Could you check a few things on this model? Use its own coordinates, in mm. Round coordinates to 2 decimals unless told otherwise and drop trailing zeros. Loops run counter-clockwise (first coordinate to the right, second up) from the corner with the lowest first, then second, coordinate; pieces in that order, holes last. Notation, with made-up numbers: M -28,28 L -12,28 A16 ccw -12,48 Z; hole C 41,-32 d4. An arc over 180 degrees is marked long. Answer in a Markdown table with one row per item.
```python
from build123d import *

# Parameters (mm, degrees)
BOSS_EXTRUDE1_DEPTH         = 2.54
F_1_4_CLEARANCE_HOLE2_D     = 6.7564
F_1_4_CLEARANCE_HOLE2_DEPTH = 8.382
F_1_4_CLEARANCE_HOLE2_TIP   = 2.029827343


with BuildPart() as part:
    # Sketch1 → Boss-Extrude1 (new body)
    with BuildSketch(Plane(origin=(0, 0, 0), x_dir=(0, 0, -1), z_dir=(1, 0, 0))):
        with BuildLine():
            Line((6.35, -2.630256121), (6.35, -152.4))
            ThreePointArc((6.35, -152.4), (0, -158.75), (-6.35, -152.4))
            Line((-6.35, -152.4), (-6.35, 0))
            ThreePointArc((-6.35, 0), (-5.866635031, 2.430039796), (-4.490128061, 4.490128061))
            Line((-4.490128061, 4.490128061), (13.470384182, 22.450640303))
            ThreePointArc((13.470384182, 22.450640303), (22.450640303, 22.450640303), (22.450640303, 13.470384182))
            Line((22.450640303, 13.470384182), (6.35, -2.630256121))
        make_face()
    extrude(amount=BOSS_EXTRUDE1_DEPTH)

    # 1/4 Clearance Hole2
    with Locations(Plane(origin=(2.54, 0, 0), x_dir=(0, 0, -1), z_dir=(1, 0, 0))):
        with Locations((0, 0), (0, -152.4), (17.960512242, 17.960512242)):
            Hole(F_1_4_CLEARANCE_HOLE2_D / 2, depth=F_1_4_CLEARANCE_HOLE2_DEPTH)
            with Locations((0, 0, -(F_1_4_CLEARANCE_HOLE2_DEPTH + F_1_4_CLEARANCE_HOLE2_TIP / 2))):  # 118° drill point
                Cone(0, F_1_4_CLEARANCE_HOLE2_D / 2, F_1_4_CLEARANCE_HOLE2_TIP, mode=Mode.SUBTRACT)


solid = part.part
```
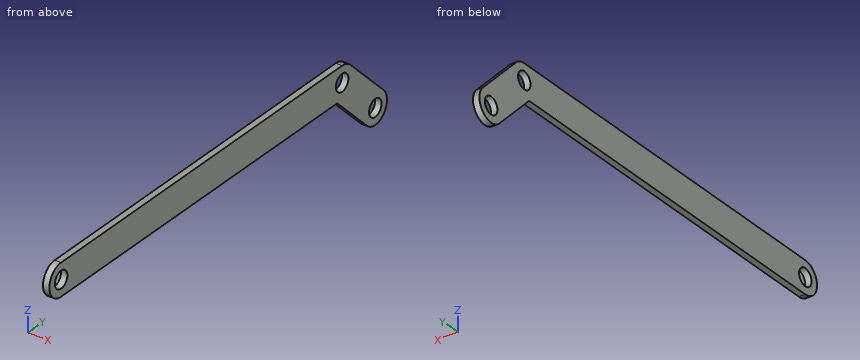
1) I want a section at C-C, the plane y = -12. Please give me the cut outline in (x, z).
Computed:
| item | result |
|---|---|
| outline | M 0,-6.35 L 2.54,-6.35 L 2.54,6.35 L 0,6.35 Z |
2) I want a section at A-A, the plane z = 0. Please give me the cut outline in (x, y).
Computed:
| item | result |
|---|---|
| outline | M 0,-158.75 L 2.54,-158.75 L 2.54,-155.78 L 0,-155.78 Z; M 0,-149.02 L 2.54,-149.02 L 2.54,-3.38 L 0,-3.38 Z; M 0,3.38 L 2.54,3.38 L 2.54,8.98 L 0,8.98 Z |
3) Will these pins go through, and if not, where does the flat tip stop? P1, Ø1.5, axis at x = 2, y = -75, coming from the -Z side; P2, Ø5.5, axis at y = -152.4, z = 0, coming from the -X side.
Computed:
| item | result |
|---|---|
| P1 | stops at z = -6.35 |
| P2 | passes through |
4) I want a section at B-B, the plane x = 0.65. Please give me the cut outline in (y, z).
Computed:
| item | result |
|---|---|
| outline | M -152.4,-6.35 L -2.63,-6.35 L 13.47,-22.45 A6.35 ccw 22.45,-13.47 L 4.49,4.49 A6.35 ccw 0,6.35 L -152.4,6.35 A6.35 ccw Z; hole C -152.4,0 d6.76; hole C 0,0 d6.76; hole C 17.96,-17.96 d6.76 |
5) I need wall thicknesses on line 1 (Z direction, x = 1.25, y = -152.4); line 2 (Y direction, x = 1.6, z = 0); line 3 (Z direction, x = 0.85, y = -138.5). Which ranges of each line are inside material? Lowest first, please.
Computed:
| item | result |
|---|---|
| line 1 | z = -6.35 to -3.38, 3.38 to 6.35 |
| line 2 | y = -158.75 to -155.78, -149.02 to -3.38, 3.38 to 8.98 |
| line 3 | z = -6.35 to 6.35 |
